```python
from build123d import *

# Parameters (mm, degrees)
PAD_DEPTH       = 3
SKETCH001_W     = 15
SKETCH001_H     = 3
POCKET_DEPTH    = 2
SKETCH002_R     = 8
PAD001_DEPTH    = 2
SKETCH003_R     = 4
POCKET001_DEPTH = 5
SKETCH004_W     = 15
SKETCH004_H     = 5
PAD002_DEPTH    = 20
POCKET002_DEPTH = 2
SKETCH006_R     = 1.5
POCKET003_DEPTH = 5
POCKET004_DEPTH = 2
SKETCH008_R     = 1.5
POCKET005_DEPTH = 5


with BuildPart() as part:
    # Sketch → Pad (new body)
    with BuildSketch(Plane.XY):
        with BuildLine():
            Line((7.5, 162), (137.5, 162))
            ThreePointArc((145, 154.5), (142.803301, 159.803301), (137.5, 162))
            Line((145, 154.5), (145, 7.5))
            ThreePointArc((137.5, 0), (142.803301, 2.196699), (145, 7.5))
            Line((137.5, 0), (7.5, 0))
            ThreePointArc((0, 7.5), (2.196699, 2.196699), (7.5, 0))
            Line((0, 7.5), (0, 154.5))
            ThreePointArc((7.5, 162), (2.196699, 159.803301), (0, 154.5))
        make_face()
    extrude(amount=PAD_DEPTH)

    # Sketch001 (on Face10 of Pad) → Pocket (cut)
    with BuildSketch(Plane.XY.offset(3)):
        with Locations((72.5, 1.5)):
            Rectangle(SKETCH001_W, SKETCH001_H)
    extrude(amount=-POCKET_DEPTH, mode=Mode.SUBTRACT)

    # Sketch002 (on Face5 of Pocket) → Pad001 (join)
    with BuildSketch(Plane.XY.offset(3)):
        with Locations((30, 110)):
            Circle(SKETCH002_R)
        with Locations((115, 110)):
            Circle(SKETCH002_R)
    extrude(amount=PAD001_DEPTH)

    # Sketch003 (on Face18 of Pad001) → Pocket001 (cut)
    with BuildSketch(Plane.XY.offset(5)):
        with Locations((30, 110)):
            Circle(SKETCH003_R)
        with Locations((115, 110)):
            Circle(SKETCH003_R)
    extrude(amount=-POCKET001_DEPTH, mode=Mode.SUBTRACT)

    # Sketch004 (on Face5 of Pocket001) → Pad002 (join)
    with BuildSketch(Plane.XY.offset(3)):
        with Locations((45, 2.5)):
            Rectangle(SKETCH004_W, SKETCH004_H)
        with Locations((100, 2.5)):
            Rectangle(SKETCH004_W, SKETCH004_H)
        with Locations((40, 159.5)):
            Rectangle(SKETCH004_W, SKETCH004_H)
        with Locations((105, 159.5)):
            Rectangle(SKETCH004_W, SKETCH004_H)
    extrude(amount=PAD002_DEPTH)

    # Sketch005 (on Face22 of Pad002) → Pocket002 (cut)
    with BuildSketch(Plane(origin=(0, 5, 0), x_dir=(-1, 0, 0), z_dir=(0, 1, 0))):
        Polygon((-98.798643, 12.375105), (-97.126096, 14.727958), (-98.327452, 17.352853), (-101.201357, 17.624895), (-102.873904, 15.272042), (-101.672548, 12.647147), align=None)
        Polygon((-43.642398, 12.452403), (-42.114915, 14.901919), (-43.472517, 17.449516), (-46.357602, 17.547597), (-47.885085, 15.098081), (-46.527483, 12.550484), align=None)
    extrude(amount=-POCKET002_DEPTH, mode=Mode.SUBTRACT)

    # Sketch006 (on Face22 of Pocket002) → Pocket003 (cut)
    with BuildSketch(Plane(origin=(0, 5, 0), x_dir=(-1, 0, 0), z_dir=(0, 1, 0))):
        with Locations((-100, 15)):
            Circle(SKETCH006_R)
        with Locations((-45, 15)):
            Circle(SKETCH006_R)
    extrude(amount=-POCKET003_DEPTH, mode=Mode.SUBTRACT)

    # Sketch007 (on Face25 of Pocket003) → Pocket004 (cut)
    with BuildSketch(Plane.XZ.offset(-157)):
        Polygon((42.303268, 13.259802), (42.65869, 16.124589), (40.355422, 17.864788), (37.696732, 16.740198), (37.34131, 13.875411), (39.644578, 12.135212), align=None)
        Polygon((106.849162, 12.783261), (107.844334, 15.493051), (105.995172, 17.709791), (103.150838, 17.216739), (102.155666, 14.506949), (104.004828, 12.290209), align=None)
    extrude(amount=-POCKET004_DEPTH, mode=Mode.SUBTRACT)

    # Sketch008 (on Face25 of Pocket004) → Pocket005 (cut)
    with BuildSketch(Plane.XZ.offset(-157)):
        with Locations((40, 15)):
            Circle(SKETCH008_R)
        with Locations((105, 15)):
            Circle(SKETCH008_R)
    extrude(amount=-POCKET005_DEPTH, mode=Mode.SUBTRACT)


solid = part.part
```
Build history of the part. All positions in model axes, mm. A direction names the side the tool comes from. Round coordinates to 2 decimals unless told otherwise and drop trailing zeros. Loops run counter-clockwise (first coordinate to the right, second up) from the corner with the lowest first, then second, coordinate; pieces in that order, holes last.
Item 1: Drill centre lines: line 1 along Z through (x, y) = (105, 161.45); line 2 along Y through (x, z) = (30, 2); line 3 along Y through (x, z) = (41.5, 12). Where is each one in solid material? Low to high.
Item 2: Saw through at A-A (y = 110). List the corners of the cut face in (x, z).
Item 3: Saw through at C-C (y = 83). List the corners of the cut face in (x, z).
Item 4: Which spindle directions (+Z, -Z, +X, -X, +Y, -Y) get a long thin tool onto all of the face, cutting with end or side? Do faces 1 (the face through (103, 157, 13)), 2 (the face through (52.5, 2, 13)), 3 (the face through (37.5, 2, 13)), 4 (the face through (47.5, 159, 13)). Say none if no direction does.
Item 5: Two-plate mould, pull along Y, no slides. Class faces 5 (the face through (92.5, 2, 13)), 6 (the face through (41.14, 159, 13.77)), 7 (the face through (72, 162, 2)): released by +Y, released by -Y, zero draft, split by the parting line, or undercut.
Item 6: Saw through at B-B (x = 115). List the corners of the cut face in (y, z).
Item 7: Pin check, flat tips, straight feed: P1, Ø9, axis at x = 30, y = 110, coming from the -Z side; P2, Ø4, axis at y = 159, z = 8, coming from the +X side; P3, Ø6.5, axis at x = 115, y = 110, coming from the -Z side; P4, Ø4, axis at y = 3, z = 11.5, coming from the -X side. Stop position of each tip, or through.
Worked answers:
1. line 1: z = 0 to 13.5, 16.5 to 23
1. line 2: y = 0 to 106, 114 to 162
1. line 3: y = 0 to 5, 157 to 162
2. outline: (0, 0) - (26, 0) - (26, 5) - (22, 5) - (22, 3) - (0, 3) - close; (34, 0) - (111, 0) - (111, 5) - (107, 5) - (107, 3) - (38, 3) - (38, 5) - (34, 5) - close; (119, 0) - (145, 0) - (145, 3) - (123, 3) - (123, 5) - (119, 5) - close
3. outline: (0, 0) - (145, 0) - (145, 3) - (0, 3) - close
4. face 1: +Z, +X, -X
4. face 2: +Z, +Y, -Y
4. face 3: +Z, -X, -Y
4. face 4: +Z, +Y
5. face 5: zero draft
5. face 6: undercut
5. face 7: released by +Y
6. outline: (0, 0) - (106, 0) - (106, 5) - (102, 5) - (102, 3) - (0, 3) - close; (114, 0) - (162, 0) - (162, 3) - (118, 3) - (118, 5) - (114, 5) - close
7. P1: stops at z = 0
7. P2: stops at x = 112.5
7. P3: passes through
7. P4: stops at x = 37.5
